from build123d import *

# Parameters (mm, degrees)
F0_W     = 200
F0_H     = 200
F1_DEPTH = 120
F3_DEPTH = 50


with BuildPart() as f1:
    # F0 (on Top) → F1 (new body)
    with BuildSketch(Plane.XY):
        Rectangle(F0_W, F0_H)
    extrude(amount=F1_DEPTH)

    # F2 (on face) → F3 (cut)
    with BuildSketch(Plane.XY.offset(120)):
        Polygon((-27.5, -12.817176), (27.5, -12.817176), (0, 34.814221), align=None)
    extrude(amount=-F3_DEPTH, mode=Mode.SUBTRACT)


solid = f1.part
The listing builds one solid part. Answer for the finished solid, in the listing's coordinates (mm). A direction names the side the tool comes from. Round coordinates to 2 decimals unless told otherwise and drop trailing zeros. Order: outer loops, then holes, each group sorted by start corner. A loop starts at its lowest first (then second) coordinate and runs counter-clockwise, first axis right, second up. Notation, with made-up numbers: M 68.25,11.5 L 87.25,11.5 A25 cw 87.25,26.5 Z; hole C 74,70.25 d5. An arc over 180 degrees is marked long. Answer in a Markdown table with one row per item. Add a question column.
1) Which of the six approach directions +Z, -Z, +X, -X, +Y, -Y give full straight-line access (tool end or side, diameter ignored) to faces 1 (the face through (-1, -21, 120)), 2 (the face through (-13.56, 11.33, 95.35))?
2) A flat-ended cylindrical pin translates along its axis: pin 1 Ø3 at (x, y) = (27, -45) entering from -Z. Find the tip coordinate at first contact, or state that the pin passes through.
3) The part is cut by section C-C on x = -9.5. Determine the outline of the cut face in (y, z), plus the area to 3 significant figures.
4) Determine the mould class of faces 3 (the face through (13.94, 10.67, 95.35)), 4 (the face through (100, -1, 59)), 5 (the face through (-1, 100, 59)), 6 (the face through (0, -12.817, 95)) for opening direction X: pulls with the +X half, pulls with the -X half, needs draft (parallel to the pull), parting line crosses it, or undercut.
5) The part is cut by section B-B on y = 6. Determine the outline of the cut face in (x, z).
6) The part is cut by section A-A on z = 77.5. Determine the outline of the cut face in (x, y), plus the area to 3 significant figures.
7) Consider line 1 along X through (y, z) = (26.5, 91.5); line 2 along Y through (x, z) = (15.5, 71.5); line 3 along X through (y, z) = (-3, 106). Determine where each line is inside the solid, lowest interval first. Write a range as from..to.
Findings below:
| question | item | result |
|---|---|---|
| 1 | face 1 | +Z, +X, -X, +Y, -Y |
| 1 | face 2 | +Z |
| 2 | pin 1 | stops at z = 0 |
| 3 | outline | M -100,0 L 100,0 L 100,120 L 18.36,120 L 18.36,70 L -12.82,70 L -12.82,120 L -100,120 Z |
| 3 | area | 22,400 mm² |
| 4 | face 3 | undercut |
| 4 | face 4 | pulls with the +X half |
| 4 | face 5 | needs draft |
| 4 | face 6 | undercut |
| 5 | outline | M -100,0 L 100,0 L 100,120 L 16.64,120 L 16.64,70 L -16.64,70 L -16.64,120 L -100,120 Z |
| 6 | outline | M -100,-100 L 100,-100 L 100,100 L -100,100 Z; hole M -27.5,-12.82 L 27.5,-12.82 L 0,34.81 Z |
| 6 | area | 38,700 mm² |
| 7 | line 1 | x = -100..-4.8, 4.8..100 |
| 7 | line 2 | y = -100..-12.82, 7.97..100 |
| 7 | line 3 | x = -100..-21.83, 21.83..100 |
